Build history of the part. All positions in model axes, mm. A direction names the side the tool comes from. Give positions to 0.01 mm unless a question says otherwise; leave off trailing zeros. Order: outer loops, then holes, each group sorted by start corner. A loop starts at its lowest first (then second) coordinate and runs counter-clockwise, first axis right, second up. Notation, with made-up numbers: (-2, 21) -> (32, 21) arc R21 ccw to (32, 48) -> close; hole circle Ø2 at (-24, 46). An arc over 180 degrees is marked (long way). One line per item, written item: value. Start each with the question number.
(1) Two-plate mould, pull along Z, no slides. Class faces 4 (the flat face through (51, 34.29, -27)), 5 (the flat face through (53, 37, -38.654)), 6 (the cylindrical face through (16.19, 3.13, 4.43)), 7 (the flat face through (51, 3, 9.606)): +Z half, -Z half, draft (parallel to the pull), parting line (faces both ways), or undercut.
(2) Which spindle directions (+Z, -Z, +X, -X, +Y, -Y) get a long thin tool onto all of the face, cutting with end or side? Do faces 1 (the cylindrical face through (15.48, 37.42, -34.32)), 2 (the flat face through (53, 24, -7.031)), 3 (the flat face through (53, 17, -15.794)). Say none if no direction does.
(3) Probe line 1 (Z direction, x = 54, y = 18); line 2 (Y direction, x = 29.5, z = -22.5); line 3 (Z direction, x = 37, y = 2). List the from-to ranges inside material, lowest first.
(4) Saw through at D-D on y = 16. Give the cut face in (x, z), plus the area to 3 significant figures.
(5) Pin check, flat tips, straight feed: pin 1 (6 mm diameter, centred on x = 65.5, y = 10, fed in from +Z); pin 2 (6.5 mm diameter, centred on x = 90.14, z = -32.3, fed in from -Y); pin 3 (6.5 mm diameter, centred on x = 13.94, z = 3.26, fed in from +Y); pin 4 (4 mm diameter, centred on x = 13.94, z = -32.3, fed in from -Y). Stop position of each tip, or through.
(6) Saw through at A-A on x = 26. Give the cut face in (y, z).
(7) Saw through at C-C on y = 3. Give the cut face in (x, z), plus the area to 3 significant figures.
(8) Saw through at B-B on z = -32. Give the cut face in (x, y), plus the area to 3 significant figures.
Autodesk Inventor part; units mm, degrees
ref_plane "YZ Plane" through (0, 0, 0) normal (1, 0, 0) x (0, 1, 0)
ref_plane "XZ Plane" through (0, 0, 0) normal (0, 1, 0) x (-1, 0, 0)
ref_plane "XY Plane" through (0, 0, 0) normal (0, 0, 1) x (1, 0, 0)
sketch "Sketch1" plane through (0, 0, 0) normal (0, 1, 0) x (-1, 0, 0)
  line L0 (11.4626, 9.6064) -> (-115.5374, 9.6064)
  line L1 (-115.5374, 9.6064) -> (-115.5374, -15.7936)
  line L2 (-115.5374, -15.7936) -> (11.4626, -15.7936)
  line L3 (11.4626, -15.7936) -> (11.4626, 9.6064)
  point P0 (0, 0)
  dimension "d0" = 25.4
  dimension "d1" = 127
extrude "Extrusion1" add sketch "Sketch1" along normal blind 6.35
sketch "Sketch2" plane through (0, 6.35, 0) normal (0, 1, 0) x (1, 0, 0)
  line L0 (115.5374, 15.7936) -> (-11.4626, 15.7936)
  line L1 (-11.4626, 15.7936) -> (-11.4626, -9.6064)
  line L2 (115.5374, -9.6064) -> (115.5374, 15.7936)
  line L3 (-11.4626, 15.7936) -> (115.5374, 15.7936)
  line L4 (115.5374, 15.7936) -> (115.5374, 3.0936)
  line L5 (115.5374, 3.0936) -> (-11.4626, 3.0936)
  line L6 (-11.4626, 3.0936) -> (-11.4626, 15.7936)
  point P0 (0, 0)
  dimension "d31" = 12.7
extrude "Extrusion2" add sketch "Sketch2" along normal blind 27.94
sketch "Sketch3" plane through (0, 34.29, 0) normal (0, 1, 0) x (1, 0, 0)
  line L0 (-11.4626, 3.0936) -> (115.5374, 3.0936)
  line L1 (-11.4626, 15.7936) -> (-11.4626, 3.0936)
  line L2 (115.5374, 15.7936) -> (-11.4626, 15.7936)
  line L3 (115.5374, 3.0936) -> (115.5374, 15.7936)
  line L4 (-11.4626, 3.0936) -> (115.5374, 3.0936)
  line L5 (115.5374, 3.0936) -> (115.5374, 38.6536)
  line L6 (115.5374, 38.6536) -> (-11.4626, 38.6536)
  line L7 (-11.4626, 38.6536) -> (-11.4626, 3.0936)
  point P0 (0, 0)
  dimension "d6" = 35.56
extrude "Extrusion3" add sketch "Sketch3" along normal blind 6.35
sketch "Sketch4" plane through (0, 40.64, 0) normal (0, 1, 0) x (1, 0, 0)
  line L0 (115.5374, 38.6536) -> (-11.4626, 38.6536)
  line L1 (-11.4626, 38.6536) -> (-11.4626, 3.0936)
  point P0 (0, 0)
  point P1 (13.9374, 32.3036)
  point P2 (90.1374, 32.3036)
  dimension "d9" = 0
  dimension "d10" = 6.35
  dimension "d11" = 76.2
  dimension "d12" = 25.4
hole "Hole1" at (13.9374, 40.64, -32.3036) at (90.1374, 40.64, -32.3036) direction (0, -1, 0) diameter 5.08 end through all
sketch "Sketch5" plane through (0, 6.35, 0) normal (0, 1, 0) x (1, 0, 0)
  line L0 (-11.4626, -9.6064) -> (115.5374, -9.6064)
  line L1 (115.5374, -9.6064) -> (115.5374, 3.0936)
  point P0 (0, 0)
  point P1 (13.9374, -3.2564)
  point P2 (90.1374, -3.2564)
  dimension "d20" = 0
  dimension "d21" = 6.35
  dimension "d22" = 25.4
  dimension "d23" = 76.2
hole "Hole2" at (13.9374, 6.35, 3.2564) at (90.1374, 6.35, 3.2564) direction (0, -1, 0) diameter 5.08 end through all
sketch "Sketch7" plane through (0, 40.64, 0) normal (0, 1, 0) x (1, 0, 0)
  line L0 (-11.4626, 3.0936) -> (115.5374, 3.0936)
  line L1 (-11.4626, 38.6536) -> (-11.4626, 3.0936)
  line L2 (115.5374, 3.0936) -> (115.5374, 38.6536)
  line L3 (-11.4626, 3.0936) -> (115.5374, 3.0936)
  line L4 (115.5374, 3.0936) -> (115.5374, 7.0306)
  line L5 (115.5374, 7.0306) -> (-11.4626, 7.0306)
  line L6 (-11.4626, 7.0306) -> (-11.4626, 3.0936)
  point P0 (0, 0)
  dimension "d35" = 3.937
extrude "Extrusion5" cut sketch "Sketch7" against normal blind 34.29
properties part number "EBoardStandoffs"
Results below:
1. face 4: draft
1. face 5: -Z half
1. face 6: undercut
1. face 7: +Z half
2. face 1: +Y, -Y
2. face 2: +Z, +X, -X, +Y
2. face 3: -Z, +X, -X, -Y
3. line 1: z = -15.79 to -7.03
3. line 2: y = 34.29 to 40.64
3. line 3: z = -15.79 to 9.61
4. outline: (-11.46, -15.79) -> (115.54, -15.79) -> (115.54, -7.03) -> (-11.46, -7.03) -> close
4. area: 1,110 mm²
5. pin 1: stops at z = -7.03
5. pin 2: stops at y = 34.29
5. pin 3: stops at y = 6.35
5. pin 4: passes through
6. outline: (0, -15.79) -> (34.29, -15.79) -> (34.29, -38.65) -> (40.64, -38.65) -> (40.64, -7.03) -> (6.35, -7.03) -> (6.35, 9.61) -> (0, 9.61) -> close
7. outline: (-11.46, -15.79) -> (115.54, -15.79) -> (115.54, 9.61) -> (-11.46, 9.61) -> close; hole circle Ø5.08 at (13.94, 3.26); hole circle Ø5.08 at (90.14, 3.26)
7. area: 3,190 mm²
8. outline: (-11.46, 34.29) -> (11.42, 34.29) -> (11.42, 40.64) -> (-11.46, 40.64) -> close; (16.46, 34.29) -> (87.62, 34.29) -> (87.62, 40.64) -> (16.46, 40.64) -> close; (92.66, 34.29) -> (115.54, 34.29) -> (115.54, 40.64) -> (92.66, 40.64) -> close
8. area: 742 mm²
